from build123d import *

# Parameters (mm, degrees)
PAD_DEPTH    = 2
SKETCH003_R  = 4
PAD001_DEPTH = 25


with BuildPart() as part:
    # Sketch → Revolution (revolve)
    with BuildSketch(Plane.XZ):
        Polygon((0, 0), (20, 0), (20, 4), (5, 16), (4, 16), (4, 18), (0, 18), align=None)
    revolve(axis=Axis((0, 0, 0), (0, 0, 1)))

    # Sketch002 (on DatumPlane) → Pad (new body)
    with BuildSketch(Plane.XY.offset(20)):
        Polygon((-3.752777, 6.5), (-7.505553, 0), (-3.752777, -6.5), (3.752777, -6.5), (7.505553, 0), (3.752777, 6.5), align=None)
    extrude(amount=-PAD_DEPTH)

    # Sketch003 (on DatumPlane) → Pad001 (join)
    with BuildSketch(Plane.XY.offset(20)):
        Circle(SKETCH003_R)
    extrude(amount=PAD001_DEPTH)


solid = part.part
Work out the finished part from the listing and answer in its coordinate system (mm). A direction names the side the tool comes from. Round coordinates to 2 decimals unless told otherwise and drop trailing zeros. Write each loop counter-clockwise with the first axis right and the second up, starting at its lowest first coordinate (ties: lowest second). Pieces come first, ordered by that corner, then holes. Notation, with made-up numbers: (-5.75, 83) - (32.25, 83) arc R27 cw to (32.25, 112) - close; hole circle Ø4 at (57, -15.75). An arc over 180 degrees is marked (long way). Answer in a Markdown table with one row per item. Add a question column.
1. The mould has two halves that part along Z. Classify faces 1 (the flat face through (3, -3, 18)), 2 (the flat face through (5.66, 3.2, 19.01)), 3 (the flat face through (3, -3, 20)): +Z half, -Z half, draft (parallel to the pull), parting line (faces both ways), or undercut.
2. A cutting plane is placed at C-C, the plane z = 22.5. Determine the outline of the cut face in (x, y).
3. Given pin 1 (10 mm diameter, centred on x = -2, z = 38.5, fed in from -Y); pin 2 (4 mm diameter, centred on y = -6.5, z = 9.5, fed in from -X); pin 3 (2 mm diameter, centred on x = 0.5, z = 19.5, fed in from +Y); pin 4 (3 mm diameter, centred on x = -12.5, z = 12.5, fed in from +Y), each flat-ended and moving along its own axis, determine where each tip first touches the part or whether it passes through.
4. A cutting plane is placed at B-B, the plane z = 13. Determine the outline of the cut face in (x, y).
5. For faces 4 (the cylindrical face through (-0.867, -3.905, 17.014)), 5 (the flat face through (5.6, -3.3, 19)), 6 (the flat face through (-5.6, 3.3, 19)), 7 (the flat face through (0, 6.5, 19)), determine the directions among +Z, -Z, +X, -X, +Y, -Y from which every point of the face is accessible in a straight line to the end or side of a thin tool.
6. A cutting plane is placed at A-A, the plane x = 0. Determine the outline of the cut face in (y, z).
7. Find the intervals of material crossed by line 1 along Z through (x, y) = (6.5, 5); line 2 along Z through (x, y) = (2, -6); line 3 along Z through (x, y) = (-10, 2.5), in increasing order. Write a range as from..to.
Worked out:
| question | item | result |
|---|---|---|
| 1 | face 1 | undercut |
| 1 | face 2 | draft |
| 1 | face 3 | +Z half |
| 2 | outline | circle Ø8 at (0, 0) |
| 3 | pin 1 | y = -4 |
| 3 | pin 2 | x = -14.34 |
| 3 | pin 3 | y = 6.5 |
| 3 | pin 4 | through |
| 4 | outline | circle Ø17.5 at (0, 0) |
| 5 | face 4 | none |
| 5 | face 5 | +Z, +X, -Y |
| 5 | face 6 | +Z, -X, +Y |
| 5 | face 7 | +Z, +X, -X, +Y |
| 6 | outline | (-20, 0) - (20, 0) - (20, 4) - (5, 16) - (4, 16) - (4, 18) - (6.5, 18) - (6.5, 20) - (4, 20) - (4, 45) - (-4, 45) - (-4, 20) - (-6.5, 20) - (-6.5, 18) - (-4, 18) - (-4, 16) - (-5, 16) - (-20, 4) - close |
| 7 | line 1 | 0..13.44 |
| 7 | line 2 | 0..14.94, 18..20 |
| 7 | line 3 | 0..11.75 |
